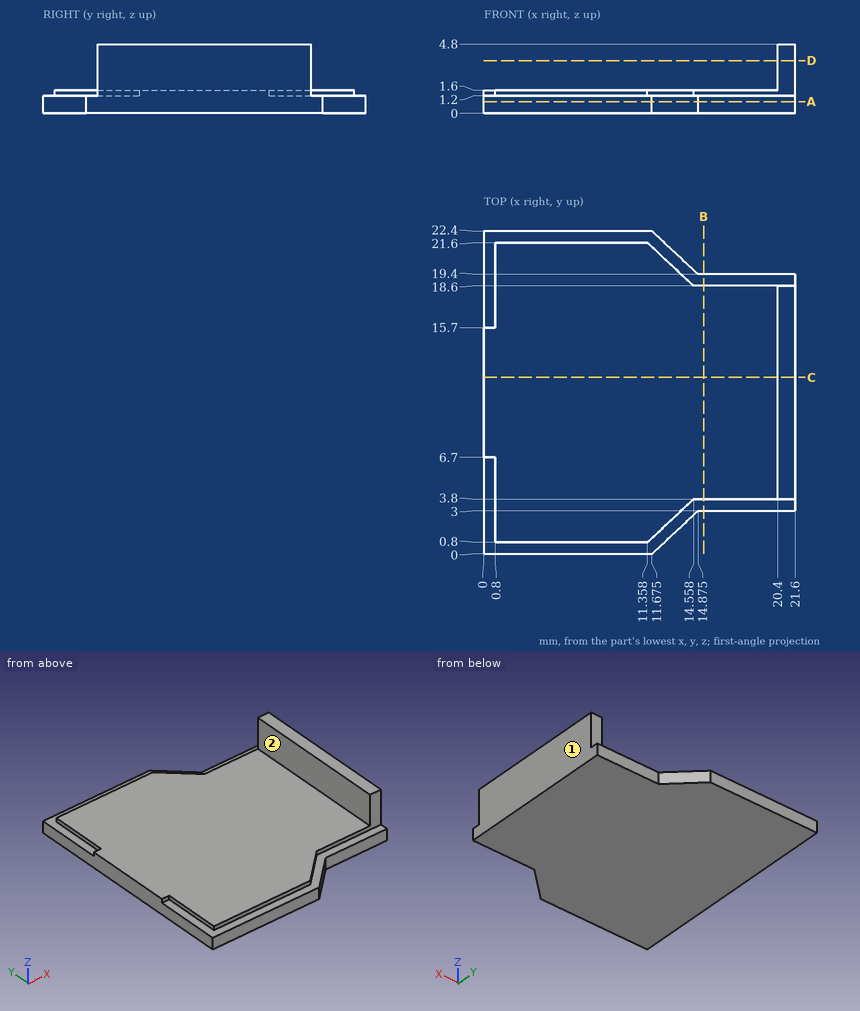
Design review of the part shown in the three views and the two pictorial views. Dimensions are in mm from the part's minimum x, y and z. A direction names the side the tool comes from. Round coordinates to 2 decimals unless told otherwise and drop trailing zeros. Write each loop counter-clockwise with the first axis right and the second up, starting at its lowest first coordinate (ties: lowest second). Pieces come first, ordered by that corner, then holes. Notation, with made-up numbers: (6.5, 80.5) -> (51.5, 80.5) arc R3 ccw to (51.5, 85.5) -> close; hole circle Ø6 at (-20.75, 67). An arc over 180 degrees is marked (long way). Write item = value, one per line. Start each with the question number.
1) Tool access review of the marked faces 1 and 2: name each direction out of +Z, -Z, +X, -X, +Y, -Y from which nothing blocks a thin tool from reaching the whole face with its end or side.
2) Clearance check with flat-ended pins moving along their axes: pin 1 (1 mm diameter, centred on x = 18, z = 1, fed in from +Y); pin 2 (1 mm diameter, centred on y = 9.5, z = 3.5, fed in from -X); pin 3 (3.5 mm diameter, centred on x = 8.5, y = 20, fed in from +Z). State where each tip first meets the part, or that it passes through.
3) Take a section at D-D, the plane z = 3.65. State the section outline as (x, y) points.
4) Take a section at C-C, the plane y = 12.25. State the section outline as (x, z) points, plus the area to 3 significant figures.
5) Take a section at A-A, the plane z = 0.8. State the section outline as (x, y) points (1 decimal).
6) Wall thickness on probe 1 along X at (y, z) = (7.25, 3.25); probe 2 along Z at (x, y) = (3.5, 14.5); probe 3 along Y at (x, z) = (20.5, 0.8): over which ranges is each line inside the solid? List them lowest first. Write a range as from..to.
7) Take a section at B-B, the plane x = 15.25. State the section outline as (y, z) points, plus the area to 3 significant figures.
Results list:
q1.face_1 = +Z, -Z, +X, +Y, -Y
q1.face_2 = +Z, -X, +Y, -Y
q2.pin_1 = 19.4
q2.pin_2 = 20.4
q2.pin_3 = 1.6
q3.outline = (20.4, 3.8) -> (21.6, 3.8) -> (21.6, 18.6) -> (20.4, 18.6) -> close
q4.outline = (0, 0) -> (21.6, 0) -> (21.6, 4.8) -> (20.4, 4.8) -> (20.4, 1.6) -> (0, 1.6) -> close
q4.area = 38.4 mm²
q5.outline = (0, 0) -> (11.7, 0) -> (14.9, 3) -> (21.6, 3) -> (21.6, 19.4) -> (14.9, 19.4) -> (11.7, 22.4) -> (0, 22.4) -> close
q6.probe_1 = 20.4..21.6
q6.probe_2 = 0..1.6
q6.probe_3 = 3..19.4
q7.outline = (3, 0) -> (19.4, 0) -> (19.4, 1.2) -> (18.6, 1.2) -> (18.6, 1.6) -> (3.8, 1.6) -> (3.8, 1.2) -> (3, 1.2) -> close
q7.area = 25.6 mm²
